Build history of the part. All positions in model axes, mm. A direction names the side the tool comes from. Round coordinates to 2 decimals unless told otherwise and drop trailing zeros. Write each loop counter-clockwise with the first axis right and the second up, starting at its lowest first coordinate (ties: lowest second). Pieces come first, ordered by that corner, then holes. Notation, with made-up numbers: (56, 63) - (78, 63) arc R6 ccw to (78, 72) - close; hole circle Ø7 at (55.5, 47). An arc over 180 degrees is marked (long way). One line per question, with ' | ' between items.
from build123d import *

# Parameters (mm, degrees)
SKETCH1_W           = 204
SKETCH1_H           = 204
SKETCH1_R           = 20
BOSS_EXTRUDE1_DEPTH = 5
SKETCH2_R           = 10
BOSS_EXTRUDE2_DEPTH = 5
BOSS_EXTRUDE3_START = 5
SKETCH3_R           = 10
SKETCH3_R_2         = 10.325688869
BOSS_EXTRUDE3_DEPTH = 5


with BuildPart() as part:
    # Sketch1 → Boss-Extrude1 (new body)
    with BuildSketch(Plane.XY):
        Rectangle(SKETCH1_W, SKETCH1_H)
        Circle(SKETCH1_R, mode=Mode.SUBTRACT)
    extrude(amount=BOSS_EXTRUDE1_DEPTH)

    # Sketch2 → Boss-Extrude2 (add)
    with BuildSketch(Plane(origin=(102, 0, 0), x_dir=(0, 0, -1), z_dir=(1, 0, 0))):
        with BuildLine():
            Line((0, 102), (-55, 102))
            Line((-55, 102), (-151.95068894, 34.723038836))
            ThreePointArc((-151.95068894, 34.723038836), (-161.540540881, 23.857555439), (-165, 9.784313725))
            Line((-165, 9.784313725), (-165, -102))
            Line((-165, -102), (-55, -102))
            Line((-55, -102), (0, -102))
            Line((0, -102), (0, 102))
        make_face()
        with Locations((-44.107183944, 78.450980392)):
            Circle(SKETCH2_R, mode=Mode.SUBTRACT)
        with Locations((-134.644967247, 9.784313725)):
            Circle(SKETCH2_R, mode=Mode.SUBTRACT)
    extrude(amount=BOSS_EXTRUDE2_DEPTH)

    # Sketch3 → Boss-Extrude3 (add)
    with BuildSketch(Plane.ZY.offset(102).offset(BOSS_EXTRUDE3_START)):
        with BuildLine():
            Line((0, 102), (0, -102))
            Line((0, -102), (165, -102))
            Line((165, -102), (165, 9.784313725))
            ThreePointArc((165, 9.784313725), (161.540540881, 23.857555439), (151.95068894, 34.723038836))
            Line((151.95068894, 34.723038836), (55, 102))
            Line((55, 102), (0, 102))
        make_face()
        with Locations(Location((44.107183944, 78.450980392, 0), (0, 0, 180))):
            Circle(SKETCH3_R, mode=Mode.SUBTRACT)
        with Locations((134.644967247, 9.784313725)):
            Circle(SKETCH3_R_2, mode=Mode.SUBTRACT)
    extrude(amount=-BOSS_EXTRUDE3_DEPTH)


solid = part.part
Q1. Saw through at C-C, the plane y = -81. List the corners of the cut face in (x, z).
Found:
outline: (-107, 0) - (107, 0) - (107, 165) - (102, 165) - (102, 5) - (-102, 5) - (-102, 165) - (-107, 165) - close
Q2. Drill centre lines: L1, parallel to X at y = 19, z = 150; L2, parallel to Y at x = 0, z = 1; L3, parallel to Z at x = -83, y = -15. Where is each one in solid material? Low to high. Write a range as from..to.
Found:
L1: -107..-102, 102..107 | L2: -102..-20, 20..102 | L3: 0..5
Q3. Drop flat-ended pins along their axis: pin 1 (18 mm diameter, centred on y = 9.78, z = 134.64, fed in from -X); pin 2 (10 mm diameter, centred on x = -58.5, y = -44, fed in from +Z); pin 3 (2 mm diameter, centred on x = -54.5, y = 1.5, fed in from -Z). Give the stop position or say it passes through.
Found:
pin 1: through | pin 2: z = 5 | pin 3: z = 0
Q4. Saw through at D-D, the plane x = 85.5. List the corners of the cut face in (y, z), then the cut area to 3 significant figures.
Found:
outline: (-102, 0) - (102, 0) - (102, 5) - (-102, 5) - close | area: 1,020 mm^2
Q5. Saw through at B-B, the plane x = 0. List the corners of the cut face in (y, z).
Found:
outline: (-102, 0) - (-20, 0) - (-20, 5) - (-102, 5) - close; (20, 0) - (102, 0) - (102, 5) - (20, 5) - close
Q6. Saw through at A-A, the plane z = 14. List the corners of the cut face in (x, y), then the cut area to 3 significant figures.
Found:
outline: (-107, -102) - (-102, -102) - (-102, 102) - (-107, 102) - close; (102, -102) - (107, -102) - (107, 102) - (102, 102) - close | area: 2,040 mm^2
Q7. Pull direction Z, two halves, no side cores. Call faces 3 (the cylindrical face through (104.465, 24.039, 161.445)), 4 (the cylindrical face through (-104.54, 10.24, 124.33)), 5 (the flat face through (-107, -21, 81)): +Z half, -Z half, draft (parallel to the pull), parting line (faces both ways), or undercut.
Found:
face 3: +Z half | face 4: undercut | face 5: draft
Q8. Which spindle directions (+Z, -Z, +X, -X, +Y, -Y) get a long thin tool onto all of the face, cutting with end or side? Do faces 1 (the flat face through (21, 1, 5)), 2 (the flat face through (0, 102, 3)). Say none if no direction does.
Found:
face 1: +Z, +Y, -Y | face 2: +Z, -Z, +X, -X, +Y
